Source: CAD feature listing. Evaluate the final solid. Frame: model axes, mm. A direction names the side the tool comes from. Round coordinates to 2 decimals unless told otherwise and drop trailing zeros. Order: outer loops, then holes, each group sorted by start corner. A loop starts at its lowest first (then second) coordinate and runs counter-clockwise, first axis right, second up. Notation, with made-up numbers: (26, 62.5) -> (64, 62.5) arc R17 cw to (64, 72.5) -> close; hole circle Ø9 at (-26.5, 62.25). An arc over 180 degrees is marked (long way). Write item = value, one per line. Start each with the question number.
(1) Cut plane A-A on y = 0. Return the cut outline in (x, z), then the cut area to 3 significant figures.
(2) Draft query along X for faces 5 (the face through (93.1, 17.99, -2.14)), 6 (the face through (90.201, -0.224, -59.434)), 7 (the face through (78.092, 15.549, 3.601)). Return one class per face: released by +X, released by -X, zero draft, split by the parting line, or undercut.
(3) Cut plane B-B on x = 80. Give the number of separate pieces and of enclosed holes in the cut face, then the cut area to 3 significant figures.
(4) Ray query, line 1 (Z direction, x = 80, y = -14.3); line 2 (Z direction, x = 80, y = -17.65); line 3 (Y direction, x = 82, z = 0). Return the intervals inside material, ascending.
(5) Contact query for flat-ended pins moving along their axis: pin 1 Ø15 at (x, y) = (10, -3) entering from -Z; pin 2 Ø4 at (x, y) = (53, -7.5) entering from -Z; pin 3 Ø1 at (y, z) = (-18.5, 6) entering from -X; pin 4 Ø3 at (x, z) = (80, 3) entering from +Y. Output: stop coordinate, or through.
(6) Reachability of faces 1 (the face through (26, 16, -17)), 2 (the face through (79, 12, 1)), 3 (the face through (47, -18, 2)), 4 (the face through (83, 15, 3)) from +Z, -Z, +X, -X, +Y, -Y: full face, straight path, thin tool, end or side. Return the list, or none.
(7) Cut plane C-C on x = 42. Return the cut outline in (y, z).
from build123d import *

# Parameters (mm, degrees)
F1_DEPTH  = 16
F2_W      = 70
F2_H      = 3
F3_DEPTH  = 2
F4_W      = 50
F4_H      = 14
F5_DEPTH  = 2
F6_R      = 1
F9_DEPTH  = 2
F11_DEPTH = 38.001
F13_D     = 4
F14_R     = 3
F14_R_2   = 2
F15_DEPTH = 5
F16_R     = 3


# Not quite as in the source:
# - a pattern or mirror of a feature is missing from the dataset's text; its kind, count and spacing are read off the source's solid


with BuildPart() as f1:
    # F0 (on Front) → F1 (new body)
    with BuildSketch(Plane.XZ):
        with BuildLine():
            Line((94, 11), (0, 11))
            ThreePointArc((0, 11), (-11, 0), (0, -11))
            Line((0, -11), (19, -11))
            ThreePointArc((19, -11), (21.7681124643, -11.8361612201), (23.6103896104, -14.064978646))
            ThreePointArc((23.6103896104, -14.064978646), (48.2280702466, -44.8445615778), (85.3629298173, -58.0511936248))
            ThreePointArc((85.3629298173, -58.0511936248), (90.2653686658, -59.4661290396), (94.3351335924, -62.5439468273))
            Line((94.3351335924, -62.5439468273), (95.6306588057, -61))
            ThreePointArc((95.6306588057, -61), (90.6542803924, -57.4351678896), (84.7034264019, -56))
            ThreePointArc((84.7034264019, -56), (49.0672193413, -42.9854179344), (25.4545454545, -13.2909701044))
            ThreePointArc((25.4545454545, -13.2909701044), (22.87535745, -10.1706257081), (19, -9))
            Line((19, -9), (0, -9))
            ThreePointArc((0, -9), (-9, 0), (0, 9))
            Line((0, 9), (94, 9))
            Line((94, 9), (94, 11))
        make_face()
    extrude(amount=F1_DEPTH)

    # F2 (on face) → F3 (join)
    with BuildSketch(Plane.XY.offset(11)):
        with Locations((59, -17.5)):
            Rectangle(F2_W, F2_H)
    extrude(amount=-F3_DEPTH)

    # F4 (on face) → F5 (join)
    with BuildSketch(Plane.XZ.offset(19)):
        with Locations((69, 4)):
            Rectangle(F4_W, F4_H)
    extrude(amount=-F5_DEPTH)

    # F6
    f6_edges = [f1.edges().sort_by_distance(p)[0] for p in [
        (59, -19, 11),
    ]]
    fillet(f6_edges, radius=F6_R)

    # F7: F1 across plane


with BuildPart() as f1_1:
    add(f1.part)
    add(f1.part.mirror(Plane.XZ))

    # F8 (on face) → F9 (cut)
    with BuildSketch(Plane.XY.offset(11)):
        with BuildLine():
            Line((94, 12), (34, 12))
            ThreePointArc((34, 12), (22.0005037904, 0.1099577956), (33.7800936413, -11.9979848805))
            Line((33.7800936413, -11.9979848805), (34.2199063587, -11.9979848805))
            Line((34.2199063587, -11.9979848805), (94, -11.9979848805))
            Line((94, -11.9979848805), (94, 12))
        make_face()
    extrude(amount=-F9_DEPTH, mode=Mode.SUBTRACT)

    # F10 (on face) → F11 (cut, through all)
    with BuildSketch(Plane.XZ.offset(19)):
        with BuildLine():
            ThreePointArc((50, 5), (47, 2), (50, -1))
            Line((50, -1), (70, -1))
            ThreePointArc((70, -1), (73, 2), (70, 5))
            Line((70, 5), (50, 5))
        make_face()
    extrude(amount=-F11_DEPTH, mode=Mode.SUBTRACT)

    # F13 (through all)
    with Locations(Plane.XZ.offset(19)):
        with Locations((80, 3)):
            Hole(F13_D / 2)

    # F14 (on face) → F15 (join)
    with BuildSketch(Plane(origin=(0, -17, 0), x_dir=(-1, 0, 0), z_dir=(0, 1, 0))):
        with Locations((-80, 3)):
            Circle(F14_R)
        with Locations((-80, 3)):
            Circle(F14_R_2, mode=Mode.SUBTRACT)
    f15 = extrude(amount=F15_DEPTH)

    # F15_copies: F15 across plane
    add(f15.mirror(Plane.ZX))

    # F16
    f16_edges = [f1_1.edges().sort_by_distance(p)[0] for p in [
        (94, -18, -3),
        (44, -18, -3),
        (44, 18, -3),
        (94, 18, -3),
    ]]
    fillet(f16_edges, radius=F16_R)


solid = f1_1.part
Evaluation:
q1.outline = (0, -11) -> (19, -11) arc R5 cw to (23.61, -14.06) arc R72 ccw to (85.36, -58.05) arc R14 cw to (94.34, -62.54) -> (95.63, -61) arc R16 ccw to (84.7, -56) arc R70 cw to (25.45, -13.29) arc R7 ccw to (19, -9) -> (0, -9) arc R9 cw to (0, 9) -> (22, 9) -> (22, 11) -> (0, 11) arc R11 ccw to start
q1.area = 338 mm^2
q2.face_5 = released by +X
q2.face_6 = released by -X
q2.face_7 = undercut
q3.separate_pieces = 5
q3.enclosed_holes = 0
q3.area = 144 mm^2
q4.line_1 = -57.5 to -55.48, 0 to 1, 5 to 6, 9 to 11
q4.line_2 = -3 to 1, 5 to 11
q4.line_3 = -19 to -17, 17 to 19
q5.pin_1 = -11
q5.pin_2 = -49.12
q5.pin_3 = 44
q5.pin_4 = through
q6.face_1 = -Z, -X, +Y
q6.face_2 = +Z, +X
q6.face_3 = +Y, -Y
q6.face_4 = none
q7.outline = (-19, 9) -> (-12, 9) -> (-12, 11) -> (-18, 11) arc R1 ccw to (-19, 10) -> close; (-16, -39.87) -> (16, -39.87) -> (16, -37.15) -> (-16, -37.15) -> close; (12, 9) -> (19, 9) -> (19, 10) arc R1 ccw to (18, 11) -> (12, 11) -> close
